from build123d import *

# Parameters (mm, degrees)
SKETCH_1_W          = 34
SKETCH_1_H          = 44
EXTRUDE_1_DEPTH     = 8
SKETCH_2_W          = 30
SKETCH_2_H          = 40
CUT_EXTRUDE_1_DEPTH = 4.5
SKETCH_3_W          = 30
SKETCH_3_H          = 30
CUT_EXTRUDE_2_DEPTH = 1.5
FILLET_1_R          = 4
CUT_EXTRUDE_3_DEPTH = 2
CUT_EXTRUDE_4_DEPTH = 1.5


with BuildPart() as part:
    # Эскиз1 → Бобышка-Вытянуть1 (new body)
    with BuildSketch(Plane.XY):
        Rectangle(SKETCH_1_W, SKETCH_1_H)
    extrude(amount=EXTRUDE_1_DEPTH)

    # Эскиз2 → Вырез-Вытянуть1 (cut)
    with BuildSketch(Plane.XY.offset(8)):
        Rectangle(SKETCH_2_W, SKETCH_2_H)
    extrude(amount=-CUT_EXTRUDE_1_DEPTH, mode=Mode.SUBTRACT)

    # Эскиз3 → Вырез-Вытянуть2 (cut)
    with BuildSketch(Plane.XY.offset(3.5)):
        with Locations((0, -5)):
            Rectangle(SKETCH_3_W, SKETCH_3_H)
    extrude(amount=-CUT_EXTRUDE_2_DEPTH, mode=Mode.SUBTRACT)

    # Скругление1
    fillet_1_edges = [part.edges().sort_by_distance(p)[0] for p in [
        (17, -22, 4),
        (-17, -22, 4),
        (-17, 22, 4),
        (17, 22, 4),
    ]]
    fillet(fillet_1_edges, radius=FILLET_1_R)

    # Эскиз4 → Вырез-Вытянуть3 (cut)
    with BuildSketch(Plane.XZ.offset(22)):
        with BuildLine():
            Line((-3, 6.5), (3, 6.5))
            ThreePointArc((3, 6.5), (4.5, 5), (3, 3.5))
            Line((3, 3.5), (-3, 3.5))
            ThreePointArc((-3, 3.5), (-4.5, 5), (-3, 6.5))
        make_face()
    extrude(amount=-CUT_EXTRUDE_3_DEPTH, mode=Mode.SUBTRACT)

    # Эскиз5 → Вырез-Вытянуть4 (cut)
    with BuildSketch(Plane.XY.offset(8)):
        with BuildLine():
            Line((-13, -21), (13, -21))
            ThreePointArc((13, -21), (15.121320344, -20.121320344), (16, -18))
            Line((16, -18), (16, 18))
            ThreePointArc((16, 18), (15.121320344, 20.121320344), (13, 21))
            Line((13, 21), (-13, 21))
            ThreePointArc((-13, 21), (-15.121320344, 20.121320344), (-16, 18))
            Line((-16, 18), (-16, -18))
            ThreePointArc((-16, -18), (-15.121320344, -20.121320344), (-13, -21))
        make_face()
    extrude(amount=-CUT_EXTRUDE_4_DEPTH, mode=Mode.SUBTRACT)


solid = part.part
Work out the finished part from the listing and answer in its coordinate system (mm). A direction names the side the tool comes from. Round coordinates to 2 decimals unless told otherwise and drop trailing zeros. Write each loop counter-clockwise with the first axis right and the second up, starting at its lowest first coordinate (ties: lowest second). Pieces come first, ordered by that corner, then holes.
1) Given pin 1 Ø15 at (x, y) = (-4, -9.5) entering from +Z; pin 2 Ø3 at (x, y) = (5.5, 14.5) entering from +Z, each flat-ended and moving along its own axis, determine where each tip first touches the part or whether it passes through.
2) The mould has two halves that part along Z. Classify faces 4 (the flat face through (-15, 0, 4)), 5 (the flat face through (0, 15, 3.5)), 6 (the flat face through (0, -21.5, 6.5)): pulls with the +Z half, pulls with the -Z half, needs draft (parallel to the pull), parting line crosses it, or undercut.
3) Straight lines are drawn through the part: line 1 (Y direction, x = 10, z = 4.5); line 2 (X direction, y = 14.5, z = 6); line 3 (Y direction, x = -13, z = 7.25). For each, find the intervals that lie inside material, in ascending order.
4) A cutting plane is placed at D-D (z = 5). Give the vertices of the cut face in (x, y).
5) A cutting plane is placed at C-C (x = 6.5). Give the vertices of the cut face in (y, z), plus the area to 3 significant figures.
6) A cutting plane is placed at B-B (y = 11.5). Give the vertices of the cut face in (x, z).
7) A cutting plane is placed at A-A (z = 7.25). Give the vertices of the cut face in (x, y), plus the area to 3 significant figures.
8) A tool of negligible diameter and unlimited length cuts with its end or side. For faces 1 (the flat face through (0, -21, 3.5)), 2 (the flat face through (0, -5, 2)), 3 (the cylindrical face through (15.859, -20.797, 4.056)), from which of +Z, -Z, +X, -X, +Y, -Y can it reach the whole face along a straight path? Write none if from no direction.
Completed:
1. pin 1: stops at z = 2
1. pin 2: stops at z = 3.5
2. face 4: needs draft
2. face 5: pulls with the +Z half
2. face 6: undercut
3. line 1: y = -22 to -20, 20 to 22
3. line 2: x = -17 to -15, 15 to 17
3. line 3: y = -22 to -21, 21 to 22
4. outline: (-17, -18) arc R4 ccw to (-13, -22) - (-4.5, -22) - (-4.5, -20) - (-15, -20) - (-15, 20) - (15, 20) - (15, -20) - (4.5, -20) - (4.5, -22) - (13, -22) arc R4 ccw to (17, -18) - (17, 18) arc R4 ccw to (13, 22) - (-13, 22) arc R4 ccw to (-17, 18) - close
5. outline: (-22, 0) - (22, 0) - (22, 8) - (21, 8) - (21, 6.5) - (20, 6.5) - (20, 3.5) - (10, 3.5) - (10, 2) - (-20, 2) - (-20, 6.5) - (-21, 6.5) - (-21, 8) - (-22, 8) - close
5. area: 124 mm2
6. outline: (-17, 0) - (17, 0) - (17, 8) - (16, 8) - (16, 6.5) - (15, 6.5) - (15, 3.5) - (-15, 3.5) - (-15, 6.5) - (-16, 6.5) - (-16, 8) - (-17, 8) - close
7. outline: (-17, -18) arc R4 ccw to (-13, -22) - (13, -22) arc R4 ccw to (17, -18) - (17, 18) arc R4 ccw to (13, 22) - (-13, 22) arc R4 ccw to (-17, 18) - close; hole (-16, -18) arc R3 ccw to (-13, -21) - (13, -21) arc R3 ccw to (16, -18) - (16, 18) arc R3 ccw to (13, 21) - (-13, 21) arc R3 ccw to (-16, 18) - close
7. area: 146 mm2
8. face 1: -Y
8. face 2: +Z
8. face 3: +Z, -Z, +X, -Y
